Build history of the part. All positions in model axes, mm. A direction names the side the tool comes from. Round coordinates to 2 decimals unless told otherwise and drop trailing zeros. Order: outer loops, then holes, each group sorted by start corner. A loop starts at its lowest first (then second) coordinate and runs counter-clockwise, first axis right, second up. Notation, with made-up numbers: (49.25, 29) - (60.25, 29) arc R24 ccw to (60.25, 46) - close; hole circle Ø5 at (37, 73). An arc over 180 degrees is marked (long way). Write each question's results on one line, items separated by ' | '. Start each with the question number.
```python
from build123d import *

# Parameters (mm, degrees)
RESSALTO_EXTRUS_O1_DEPTH = 5
ESBO_O2_R                = 1.5
CORTE_EXTRUS_O1_DEPTH    = 5
ESBO_O3_R                = 1.5
CORTE_EXTRUS_O2_DEPTH    = 10
CORTE_EXTRUS_O3_DEPTH    = 10


with BuildPart() as part:
    # Esboço1 → Ressalto-extrusão1 (new body)
    with BuildSketch(Plane(origin=(0, 0, 0), x_dir=(1, 0, 0), z_dir=(0, 1, 0))):
        with BuildLine():
            Line((-61.865783789, 131.661644013), (109.134216211, 131.661644013))
            ThreePointArc((109.134216211, 131.661644013), (112.669750117, 130.197177919), (114.134216211, 126.661644013))
            Line((114.134216211, 126.661644013), (114.134216211, -23.338355987))
            ThreePointArc((114.134216211, -23.338355987), (112.669750117, -26.873889893), (109.134216211, -28.338355987))
            Line((109.134216211, -28.338355987), (-61.865783789, -28.338355987))
            ThreePointArc((-61.865783789, -28.338355987), (-65.401317695, -26.873889893), (-66.865783789, -23.338355987))
            Line((-66.865783789, -23.338355987), (-66.865783789, 126.661644013))
            ThreePointArc((-66.865783789, 126.661644013), (-65.401317695, 130.197177919), (-61.865783789, 131.661644013))
        make_face()
    extrude(amount=RESSALTO_EXTRUS_O1_DEPTH)

    # Esboço2 → Corte-extrusão1 (cut)
    with BuildSketch(Plane(origin=(0, 5, 0), x_dir=(1, 0, 0), z_dir=(0, 1, 0))):
        with Locations(Location((-27.865783789, 98.161644013, 0), (0, 0, 270))):
            Circle(ESBO_O2_R)
        with Locations(Location((75.134216211, 98.161644013, 0), (0, 0, 270))):
            Circle(ESBO_O2_R)
        with Locations(Location((-8.115783789, 4.161644013, 0), (0, 0, 270))):
            Circle(ESBO_O2_R)
        with Locations(Location((55.384216211, 4.161644013, 0), (0, 0, 270))):
            Circle(ESBO_O2_R)
    extrude(amount=-CORTE_EXTRUS_O1_DEPTH, mode=Mode.SUBTRACT)

    # Esboço3 → Corte-extrusão2 (cut)
    with BuildSketch(Plane(origin=(0, 5, 0), x_dir=(1, 0, 0), z_dir=(0, 1, 0))):
        with Locations(Location((-39.865783789, 46.661644013, 0), (0, 0, 270))):
            Circle(ESBO_O3_R)
        with Locations(Location((-39.865783789, 4.611644013, 0), (0, 0, 270))):
            Circle(ESBO_O3_R)
        with Locations(Location((87.134216211, 46.661644013, 0), (0, 0, 270))):
            Circle(ESBO_O3_R)
        with Locations(Location((87.134216211, 4.611644013, 0), (0, 0, 270))):
            Circle(ESBO_O3_R)
    extrude(amount=-CORTE_EXTRUS_O2_DEPTH, mode=Mode.SUBTRACT)

    # Esboço4 → Corte-extrusão3 (cut)
    with BuildSketch(Plane(origin=(0, 5, 0), x_dir=(1, 0, 0), z_dir=(0, 1, 0))):
        with BuildLine():
            Line((-4.365783789, 62.661644013), (51.634216211, 62.661644013))
            ThreePointArc((51.634216211, 62.661644013), (53.401983164, 61.929410966), (54.134216211, 60.161644013))
            Line((54.134216211, 60.161644013), (54.134216211, 50.161644013))
            ThreePointArc((54.134216211, 50.161644013), (53.401983164, 48.39387706), (51.634216211, 47.661644013))
            Line((51.634216211, 47.661644013), (-4.365783789, 47.661644013))
            ThreePointArc((-4.365783789, 47.661644013), (-6.133550742, 48.39387706), (-6.865783789, 50.161644013))
            Line((-6.865783789, 50.161644013), (-6.865783789, 60.161644013))
            ThreePointArc((-6.865783789, 60.161644013), (-6.133550742, 61.929410966), (-4.365783789, 62.661644013))
        make_face()
    extrude(amount=-CORTE_EXTRUS_O3_DEPTH, mode=Mode.SUBTRACT)


solid = part.part
```
1. Cut at A-A (x = 27). List the corners of the cut face in (y, z).
2. Flat gauge pins, fed straight in: pin 1 Ø1.8 at (x, z) = (-39.87, -46.66) entering from -Y; pin 2 Ø5 at (x, z) = (87.13, -4.61) entering from -Y. Where does each tip first touch, or does it go through?
3. Mould opens along X. For faces 1 (the face through (-66.866, 2, -51)), 2 (the face through (24, 3, -47.662)), 3 (the face through (25, 5, -71)) say: pulls with the +X half, pulls with the -X half, needs draft (parallel to the pull), parting line crosses it, or undercut.
4. Wall check: line 1 (Z direction, x = 44, y = 3.2); line 2 (X direction, y = 2, z = -5). Give the ranges that are in metal, low to high. Write a range as from..to.
5. 3-axis set-ups, long thin cutter, end or side, ignore diameter. For faces 4 (the face through (-6.866, 3, -55)), 5 (the face through (-65.4, 2.5, -130.2)): which of +Z, -Z, +X, -X, +Y, -Y reach the whole face in a straight line?
6. Cut at B-B (y = 3.6). Give the number of separate pieces and of enclosed holes in the cut face, plus the area to 3 significant figures.
A:
1) outline: (0, -131.66) - (5, -131.66) - (5, -62.66) - (0, -62.66) - close; (0, -47.66) - (5, -47.66) - (5, 28.34) - (0, 28.34) - close
2) pin 1: passes through | pin 2: stops at y = 0
3) face 1: pulls with the -X half | face 2: undercut | face 3: needs draft
4) line 1: z = -131.66..-62.66, -47.66..28.34 | line 2: x = -66.87..-41.31, -38.42..-9.36, -6.87..54.14, 56.63..85.69, 88.58..114.13
5) face 4: +Y, -Y | face 5: -Z, -X, +Y, -Y
6) separate pieces: 1 | enclosed holes: 9 | area: 28,000 mm^2
